Input: part model. Units: mm. Frame: model coordinates. A direction names the side the tool comes from. Give positions to 0.01 mm unless a question says otherwise; leave off trailing zeros. Loops run counter-clockwise (first coordinate to the right, second up) from the corner with the lowest first, then second, coordinate; pieces in that order, holes last. Notation, with made-up numbers: M -9,39.25 L 39,39.25 A20 ccw 39,61.25 Z; hole C 31.5,0.25 d9. An arc over 180 degrees is marked long. Use CSV: the item, a comma, the result in double quotes. Start each with the question number.
from build123d import *

# Parameters (mm, degrees)
SKETCH_1_W          = 40
SKETCH_1_H          = 15
EXTRUDE_1_DEPTH     = 6
SKETCH_2_W          = 31.7
SKETCH_2_H          = 11.25
EXTRUDE_2_DEPTH     = 4
EXTRUDE_3_DEPTH     = 3
SKETCH_4_W          = 20
SKETCH_4_H          = 1
SKETCH_4_H_2        = 2.25
CUT_EXTRUDE_1_DEPTH = 1
SKETCH_6_R          = 1.05
CUT_EXTRUDE_2_DEPTH = 24.178653973
SKETCH_7_R          = 2
CUT_EXTRUDE_3_DEPTH = 2.1
SKETCH_8_R          = 1.25
CUT_EXTRUDE_4_DEPTH = 24.58495283
SKETCH_9_R          = 2.5
EXTRUDE_4_DEPTH     = 10
SKETCH_10_R         = 0.8
CUT_EXTRUDE_5_DEPTH = 26.739075352
CUT_EXTRUDE_6_DEPTH = 1
SKETCH_13_R         = 2.75
CUT_EXTRUDE_8_DEPTH = 3.1


with BuildPart() as part:
    # 草图1 → 凸台-拉伸1 (new body)
    with BuildSketch(Plane(origin=(0, 0, 0), x_dir=(1, 0, 0), z_dir=(0, 1, 0))):
        Rectangle(SKETCH_1_W, SKETCH_1_H)
    extrude(amount=EXTRUDE_1_DEPTH)

    # 草图2 → 凸台-拉伸2 (add)
    with BuildSketch(Plane(origin=(0, 6, 0), x_dir=(1, 0, 0), z_dir=(0, 1, 0))):
        with Locations((4.15, -1.875)):
            Rectangle(SKETCH_2_W, SKETCH_2_H)
        with BuildLine():
            Line((-6.7, 2.75), (16.3, 2.75))
            ThreePointArc((16.3, 2.75), (17.007106781, 2.457106781), (17.3, 1.75))
            Line((17.3, 1.75), (17.3, -4.25))
            ThreePointArc((17.3, -4.25), (17.007106781, -4.957106781), (16.3, -5.25))
            Line((16.3, -5.25), (-6.7, -5.25))
            ThreePointArc((-6.7, -5.25), (-7.407106781, -4.957106781), (-7.7, -4.25))
            Line((-7.7, -4.25), (-7.7, 1.75))
            ThreePointArc((-7.7, 1.75), (-7.407106781, 2.457106781), (-6.7, 2.75))
        make_face(mode=Mode.SUBTRACT)
    extrude(amount=EXTRUDE_2_DEPTH)

    # 草图3 → 凸台-拉伸3 (add)
    with BuildSketch(Plane(origin=(0, 6, 0), x_dir=(1, 0, 0), z_dir=(0, 1, 0))):
        with BuildLine():
            Line((-6.7, -5.25), (16.3, -5.25))
            ThreePointArc((16.3, -5.25), (17.007106781, -4.957106781), (17.3, -4.25))
            Line((17.3, -4.25), (17.3, 1.75))
            ThreePointArc((17.3, 1.75), (17.007106781, 2.457106781), (16.3, 2.75))
            Line((16.3, 2.75), (-6.7, 2.75))
            ThreePointArc((-6.7, 2.75), (-7.407106781, 2.457106781), (-7.7, 1.75))
            Line((-7.7, 1.75), (-7.7, -4.25))
            ThreePointArc((-7.7, -4.25), (-7.407106781, -4.957106781), (-6.7, -5.25))
        make_face()
    extrude(amount=EXTRUDE_3_DEPTH)

    # 草图4 → 切除-拉伸1 (cut)
    with BuildSketch(Plane(origin=(0, 10, 0), x_dir=(1, 0, 0), z_dir=(0, 1, 0))):
        with Locations((4.8, 3.25)):
            Rectangle(SKETCH_4_W, SKETCH_4_H)
        with Locations((4.8, -6.375)):
            Rectangle(SKETCH_4_W, SKETCH_4_H_2)
    extrude(amount=-CUT_EXTRUDE_1_DEPTH, mode=Mode.SUBTRACT)

    # 草图6 → 切除-拉伸2 (cut, through all)
    with BuildSketch(Plane(origin=(0, 9, 0), x_dir=(1, 0, 0), z_dir=(0, 1, 0))):
        with Locations(Location((-5.7, -1.25, 0), (0, 0, 270))):
            Circle(SKETCH_6_R)
        with Locations(Location((15.3, -1.25, 0), (0, 0, 90))):
            Circle(SKETCH_6_R)
    extrude(amount=-CUT_EXTRUDE_2_DEPTH, mode=Mode.SUBTRACT)

    # 草图7 → 切除-拉伸3 (cut)
    with BuildSketch(Plane.XZ):
        with Locations(Location((-5.7, 1.25, 0), (0, 0, 270))):
            Circle(SKETCH_7_R)
        with Locations(Location((15.3, 1.25, 0), (0, 0, 270))):
            Circle(SKETCH_7_R)
    extrude(amount=-CUT_EXTRUDE_3_DEPTH, mode=Mode.SUBTRACT)

    # 草图8 → 切除-拉伸4 (cut, through all)
    with BuildSketch(Plane.XZ):
        with Locations(Location((-15, 2.5, 0), (0, 0, 270))):
            Circle(SKETCH_8_R)
        with Locations(Location((5, 2.5, 0), (0, 0, 270))):
            Circle(SKETCH_8_R)
    extrude(amount=-CUT_EXTRUDE_4_DEPTH, mode=Mode.SUBTRACT)

    # 草图9 → 凸台-拉伸4 (add)
    with BuildSketch(Plane(origin=(0, 0, 0), x_dir=(1, 0, 0), z_dir=(0, 1, 0))):
        with Locations((20, -1.875)):
            Circle(SKETCH_9_R)
        with Locations((-10.4, -1.875)):
            Circle(SKETCH_9_R)
    extrude(amount=EXTRUDE_4_DEPTH)

    # 草图10 → 切除-拉伸5 (cut, through all)
    with BuildSketch(Plane(origin=(0, 10, 0), x_dir=(1, 0, 0), z_dir=(0, 1, 0))):
        with Locations(Location((-10.4, -1.875, 0), (0, 0, 270))):
            Circle(SKETCH_10_R)
        with Locations(Location((20, -1.875, 0), (0, 0, 270))):
            Circle(SKETCH_10_R)
    extrude(amount=-CUT_EXTRUDE_5_DEPTH, mode=Mode.SUBTRACT)

    # 草图11 → 切除-拉伸6 (cut)
    with BuildSketch(Plane(origin=(0, 10, 0), x_dir=(1, 0, 0), z_dir=(0, 1, 0))):
        with BuildLine():
            Line((17.4, 1.75), (17.4, -4.25))
            ThreePointArc((17.4, -4.25), (17.077817459, -5.027817459), (16.3, -5.35))
            Line((16.3, -5.35), (-6.7, -5.35))
            ThreePointArc((-6.7, -5.35), (-7.477817459, -5.027817459), (-7.8, -4.25))
            Line((-7.8, -4.25), (-7.8, 1.75))
            ThreePointArc((-7.8, 1.75), (-7.477817459, 2.527817459), (-6.7, 2.85))
            Line((-6.7, 2.85), (16.3, 2.85))
            ThreePointArc((16.3, 2.85), (17.077817459, 2.527817459), (17.4, 1.75))
        make_face()
    extrude(amount=-CUT_EXTRUDE_6_DEPTH, mode=Mode.SUBTRACT)

    # 草图13 → 切除-拉伸8 (cut)
    with BuildSketch(Plane.XZ):
        with Locations(Location((-15, -4.5, 0), (0, 0, 270))):
            Circle(SKETCH_13_R)
        with Locations(Location((-5, -4.5, 0), (0, 0, 270))):
            Circle(SKETCH_13_R)
        with Locations(Location((5, -4.5, 0), (0, 0, 270))):
            Circle(SKETCH_13_R)
        with Locations(Location((15, -4.5, 0), (0, 0, 270))):
            Circle(SKETCH_13_R)
    extrude(amount=-CUT_EXTRUDE_8_DEPTH, mode=Mode.SUBTRACT)


solid = part.part
Item 1: Material intervals for line 1 (X direction, y = 2.3, z = -4.5); line 2 (X direction, y = 0.5, z = -2.25); line 3 (Z direction, x = -10.5, y = 3), sorted ascending.
Item 2: First-contact query: pin 1 Ø6 at (x, z) = (15.5, -4) entering from -Y; pin 2 Ø3.5 at (x, z) = (-15, -4.5) entering from -Y; pin 3 Ø2 at (x, z) = (-6, 1.5) entering from -Y; pin 4 Ø1.2 at (x, y) = (1, 7.5) entering from -Z. Flat tips, straight axial feed; report the tip coordinate or a pass-through.
Item 3: Section C-C (y = 8). Output: boundary loops of the cut face in (x, z) (3 decimals), then the cut area to 3 significant figures.
Item 4: Mould query, pull axis Z, two halves, no side actions, for faces 1 (the cylindrical face through (-4.66, 5.6, 1.11)), 2 (the flat face through (-20, 3, 0)). Classes: +Z half, -Z half, draft (parallel to the pull), parting line (faces both ways), or undercut.
Item 5: Section A-A (x = 5). Output: boundary loops of the cut face in (y, z), then the cut area to 3 significant figures.
Item 6: Section B-B (y = 1.5). State how many separate pieces and enclosed holes the cut face has, then the cut area to 3 significant figures.
Item 7: Section D-D (z = -4.25). Output: boundary loops of the cut face in (x, y), then the cut area to 3 significant figures.
Item 8: Set-up query: faces 3 (the flat face through (20, 5, 6)), 4 (the flat face through (15.6, 9.5, 5.35)), 5 (the cylindrical face through (-12.68, 1.53, -5.98)), 6 (the flat face through (-5.2, 9.5, 6.4)). Return all of +Z, -Z, +X, -X, +Y, -Y with unobstructed straight access to the full face (end or side cutting, diameter ignored); none if empty.
Recorded:
1,line 1,"-20 to -17.75, -12.25 to -7.75, -2.25 to 2.25, 7.75 to 12.25, 17.75 to 20"
1,line 2,"-20 to -16.58, -13.42 to -6.58, -3.42 to 3.42, 6.58 to 13.42, 16.58 to 20"
1,line 3,"-7.5 to 1.08, 2.67 to 7.5"
2,pin 1,"y = 0"
2,pin 2,"y = 3.1"
2,pin 3,"y = 2.1"
2,pin 4,"z = -3.75"
3,outline,"M -11.7,-3.75 L 20,-3.75 L 20,-0.625 A2.5 ccw 20,4.375 L 20,7.5 L -11.7,7.5 L -11.7,4.01 A2.5 ccw -11.7,-0.26 Z; hole C -10.4,1.875 d1.6; hole C -5.7,1.25 d2.1; hole C 5,2.5 d2.5; hole C 15.3,1.25 d2.1; hole C 20,1.875 d1.6"
3,area,"354 mm²"
4,face 1,"undercut"
4,face 2,"draft"
5,outline,"M 0,-7.5 L 6,-7.5 L 6,-3.75 L 9,-3.75 L 9,1.25 L 0,1.25 L 0,-1.75 L 3.1,-1.75 L 3.1,-7.25 L 0,-7.25 Z; M 0,3.75 L 9,3.75 L 9,7.5 L 0,7.5 Z"
5,area,"84.2 mm²"
6,separate pieces,"1"
6,enclosed holes,"10"
6,area,"476 mm²"
7,outline,"M -20,0 L -17.74,0 L -17.74,3.1 L -12.26,3.1 L -12.26,0 L -7.74,0 L -7.74,3.1 L -2.26,3.1 L -2.26,0 L 2.26,0 L 2.26,3.1 L 7.74,3.1 L 7.74,0 L 12.26,0 L 12.26,3.1 L 17.74,3.1 L 17.74,0 L 20,0 L 20,6 L -20,6 Z"
7,area,"172 mm²"
8,face 3,"+Z, +X, +Y, -Y"
8,face 4,"+Y"
8,face 5,"-Y"
8,face 6,"+Z, -Z, +Y"
